Verification items for this drawing (mm, ordinates from the low corner). A direction names the side the tool comes from. Coordinates: 2 decimals unless noted, no trailing zeros. Order: outer loops, then holes, each group sorted by start corner. A loop starts at its lowest first (then second) coordinate and runs counter-clockwise, first axis right, second up. Notation, with made-up numbers: M 45,-28.75 L 64,-28.75 A27 cw 64,5.25 Z; hole C 18.25,24 d6. An arc over 180 degrees is marked long. Answer as a JSON object with one key per item and string values. Group by question number.
(1) Gauge pin test, flat ends, axial feed: pin 1 Ø3 at (x, z) = (21, 31.5) entering from -Y; pin 2 Ø4.5 at (x, z) = (19, 37.5) entering from -Y; pin 3 Ø3.5 at (x, z) = (18, 36.65) entering from +Y; pin 4 Ø0.9 at (x, y) = (4, 4.5) entering from +Z. Record the tip position at first contact, or that the pin passes through.
(2) Cross-section at D-D (x = 3.5). Enter the section's corners in (y, z), plus the area to 3 significant figures.
(3) Access from +Z, -Z, +X, -X, +Y, -Y to the whole of each face (thin tool, end or side, straight path). Record for the marked faces 1, 2 and 3.
(4) Material ranges on line 1 (Z direction, x = 8, y = 7) (3 decimals); line 2 (X direction, y = 2, z = 3) (3 decimals); line 3 (X direction, y = 3.6, z = 36.65) (3 decimals), recorded low to high.
(5) Cross-section at C-C (z = 27.5). Enter the section's corners in (x, y) (3 decimals), plus the area to 3 significant figures.
(6) Cross-section at B-B (z = 3.45). Enter the section's corners in (x, y) (3 decimals), plus the area to 3 significant figures.
(7) Cross-section at A-A (x = 18). Enter the section's corners in (y, z) (3 decimals), plus the area to 3 significant figures.
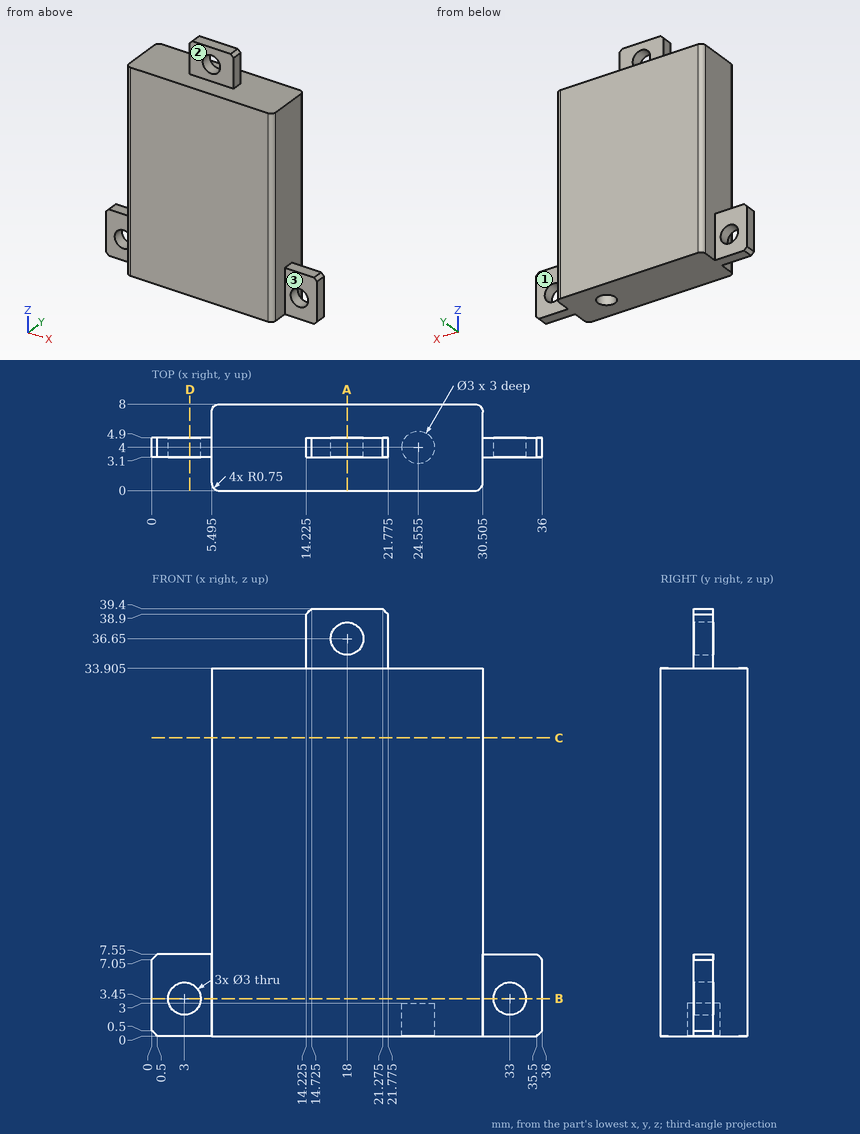
Taken from the geometry:
{
 "1": {"pin 1": "stops at y = 0", "pin 2": "stops at y = 3.1", "pin 3": "stops at y = 4.9", "pin 4": "stops at z = 7.55"},
 "2": {"outline": "M 3.1,0 L 4.9,0 L 4.9,2.04 L 3.1,2.04 Z; M 3.1,4.86 L 4.9,4.86 L 4.9,7.55 L 3.1,7.55 Z", "area": "8.50 mm²"},
 "3": {"face 1": "+Z, -Z, +X, +Y", "face 2": "+Z, +X, -X, -Y", "face 3": "+Z, -Z, +X, -Y"},
 "4": {"line 1": "z = 0 to 33.905", "line 2": "x = 5.495 to 30.505", "line 3": "x = 14.225 to 16.5, 19.5 to 21.775"},
 "5": {"outline": "M 5.495,0.75 A0.75 ccw 6.245,0 L 29.755,0 A0.75 ccw 30.505,0.75 L 30.505,7.25 A0.75 ccw 29.755,8 L 6.245,8 A0.75 ccw 5.495,7.25 Z", "area": "200 mm²"},
 "6": {"outline": "M 0,3.1 L 1.5,3.1 L 1.5,4.9 L 0,4.9 Z; M 4.5,3.1 L 5.495,3.1 L 5.495,0.75 A0.75 ccw 6.245,0 L 29.755,0 A0.75 ccw 30.505,0.75 L 30.505,3.1 L 31.5,3.1 L 31.5,4.9 L 30.505,4.9 L 30.505,7.25 A0.75 ccw 29.755,8 L 6.245,8 A0.75 ccw 5.495,7.25 L 5.495,4.9 L 4.5,4.9 Z; M 34.5,3.1 L 36,3.1 L 36,4.9 L 34.5,4.9 Z", "area": "209 mm²"},
 "7": {"outline": "M 0,0 L 8,0 L 8,33.905 L 4.9,33.905 L 4.9,35.15 L 3.1,35.15 L 3.1,33.905 L 0,33.905 Z; M 3.1,38.15 L 4.9,38.15 L 4.9,39.4 L 3.1,39.4 Z", "area": "276 mm²"}
}
